Build history of the part. All positions in model axes, mm. Give positions to 0.01 mm unless a question says otherwise; leave off trailing zeros. Loops run counter-clockwise (first coordinate to the right, second up) from the corner with the lowest first, then second, coordinate; pieces in that order, holes last. Notation, with made-up numbers: (-21, 89) -> (24, 89) arc R31 ccw to (24, 125) -> close; hole circle Ø7 at (66.25, 41). An arc over 180 degrees is marked (long way). Answer as a JSON object with one key per item and string values. Group by question number.
Q1. Drop flat-ended pins along their axis: pin 1 (1 mm diameter, centred on x = -1, z = 2, fed in from -Y); pin 2 (1 mm diameter, centred on x = -2, y = 3.5, fed in from -Z). Give the stop position or say it passes through.
Q2. Band-saw the part on C-C, the plane z = 3.45. Write the cut outline in (x, y).
Q3. Two-plate mould, pull along X, no slides. Class faces 1 (the flat face through (2, -2, 2)), 2 (the cylindrical face through (0, -2, 3)), 3 (the cylindrical face through (-0.54, -2.44, 3.97)): pulls with the +X half, pulls with the -X half, needs draft (parallel to the pull), parting line crosses it, or undercut.
Q4. Wall check: probe 1 along Y at (x, z) = (0, 4.7); probe 2 along Z at (x, y) = (0, 3); probe 3 along Y at (x, z) = (0, 1.3). Give the ranges that are in metal, low to high. Write a range as from..to.
from build123d import *

# Parameters (mm, degrees)
F0_R     = 5
F0_R_2   = 2
F2_DEPTH = 2
F3_R     = 2.5
F3_R_2   = 2
F4_DEPTH = 4
F5_R     = 1.99999


# Not quite as in the source:
# - a fillet or chamfer is up to 0.001 mm smaller than in the source, because OpenCascade refuses the exact size


with BuildPart() as f2:
    # F0 (on Top) → F2 (new body)
    with BuildSketch(Plane.XY):
        Circle(F0_R)
        Circle(F0_R_2, mode=Mode.SUBTRACT)
    extrude(amount=F2_DEPTH)

    # F3 (on face) → F4 (join)
    with BuildSketch(Plane.XY.offset(2)):
        Circle(F3_R)
        Circle(F3_R_2, mode=Mode.SUBTRACT)
    extrude(amount=F4_DEPTH)

    # F5 (radius 2 in the source; OpenCascade refuses exactly that, so slightly less here)
    f5_edges = [f2.edges().sort_by_distance(p)[0] for p in [
        (-5, 0, 0),
    ]]
    fillet(f5_edges, radius=F5_R)


solid = f2.part
Worked answers:
{
 "1": {"pin 1": "y = -4.97", "pin 2": "z = 0.07"},
 "2": {"outline": "circle Ø5 at (0, 0); hole circle Ø4 at (0, 0)"},
 "3": {"face 1": "needs draft", "face 2": "undercut", "face 3": "parting line crosses it"},
 "4": {"probe 1": "-2.5..-2, 2..2.5", "probe 2": "0..2", "probe 3": "-4.87..-2, 2..4.87"}
}
